Here's how the part is built. I have some questions about the finished solid (model axes, mm). A direction names the side the tool comes from. Coordinates: 2 decimals unless noted, no trailing zeros. Write each loop counter-clockwise with the first axis right and the second up, starting at its lowest first coordinate (ties: lowest second). Pieces come first, ordered by that corner, then holes. Notation, with made-up numbers: (31, -1.5) -> (88, -1.5) arc R4 cw to (88, 4.5) -> close; hole circle Ø1 at (-3, 10.25). An arc over 180 degrees is marked (long way). Use a Markdown table: item, result. Add a question column.
```python
from build123d import *

# Parameters (mm, degrees)
F1_DEPTH    = 6.35
F3_DEPTH    = 38.1
F4_R        = 5.08
F5_T1_DEPTH = 52.07
F5_S5_W     = 5.08
F5_S5_H     = 5.08
F5_T6_DEPTH = 5.08


# Not quite as in the source:
# - a fillet or chamfer that OpenCascade refuses, or shapes differently, is made with other operations: its cross-section is extruded or revolved along the edge and cut away or added


with BuildPart() as f1:
    # F0 (on Top) → F1 (new body)
    with BuildSketch(Plane.XY):
        Polygon((69.2906975746, 0), (0, 0), (0, -69.8406398296), (38.6781543493, -69.8406398296), (38.6781543493, -35.7452183962), (69.2906975746, -35.7452183962), align=None)
    extrude(amount=F1_DEPTH)

    # F2 (on face) → F3 (join)
    with BuildSketch(Plane(origin=(0, 0, 0), x_dir=(1, 0, 0), z_dir=(0, 0, -1))):
        Polygon((5.08, 69.8406398296), (0, 69.8406398296), (0, 0), (69.2906975746, 0), (69.2906975746, 5.08), (5.08, 5.08), align=None)
    extrude(amount=F3_DEPTH)

    # F4
    f4_edges = [f1.edges().sort_by_distance(p)[0] for p in [
        (34.645349, 0, 6.35),
        (0, -34.92032, 6.35),
        (19.339077, -69.84064, 6.35),
        (38.678154, -52.792929, 6.35),
        (53.984426, -35.745218, 6.35),
        (69.290698, -17.872609, 6.35),
    ]]
    fillet(f4_edges, radius=F4_R)

    # F5: fillet of radius 5.08 on 1 edges, made by hand

    # F5_s2 → F5_t1 (cut)
    with BuildSketch(Plane.XY.offset(-50.8)):
        with BuildLine():
            ThreePointArc((5.08, 0), (1.4878975516, -1.4878975516), (0, -5.08))
            Line((0, -5.08), (0, 0))
            Line((0, 0), (5.08, 0))
        make_face()
    extrude(amount=F5_T1_DEPTH, mode=Mode.SUBTRACT)


with BuildPart() as f5_tool4:
    # F5_s5 → F5_t6 (new body)
    with BuildSketch(Plane.XZ.offset(5.08)):
        with Locations((2.54, 3.81)):
            Rectangle(F5_S5_W, F5_S5_H)
    extrude(amount=-F5_T6_DEPTH)

    # F5_s7 → F5_t8 (revolve, cut)
    with BuildSketch(Plane(origin=(5.08, -5.08, 1.27), x_dir=(0.7071067812, 0, -0.7071067812), z_dir=(0.7071067812, 0, 0.7071067812))):
        with BuildLine():
            ThreePointArc((0, -5.08), (5.08, 0), (0, 5.08))
            Line((0, 5.08), (0, -5.08))
        make_face()
    revolve(axis=Axis((5.08, -5.08, 1.27), (0, 1, 0)), mode=Mode.SUBTRACT)


with BuildPart() as f1_1:
    add(f1.part)

    # F5_t3: cut F5_tool4
    add(f5_tool4.part, mode=Mode.SUBTRACT)


solid = f1_1.part
```
Q1. Will these pins go through, and if not, where does the flat tip stop? pin 1 (19 mm diameter, centred on x = 36, z = -26.5, fed in from -Y); pin 2 (6 mm diameter, centred on y = -26, z = -17.5, fed in from -X); pin 3 (0.6 mm diameter, centred on x = 53.5, z = 1, fed in from -Y); pin 4 (19 mm diameter, centred on y = -52, z = -14.5, fed in from +X).
Q2. Suppose I cut it at C-C, the plane z = -10. Write out the boundary of the cut face in (x, y).
Q3. Suppose I cut it at D-D, the plane x = 37.5. Write out the boundary of the cut face in (y, z).
Q4. Suppose I cut it at B-B, the plane x = 6.5. Write out the boundary of the cut face in (y, z), and give its area (3 significant figures).
Q5. Which directions (+Z, -Z, +X, -X, +Y, -Y) give clear straight access to the entire face, cutting with the end or side of a thin tool? Please do faces 1 (the cylindrical face through (37.23, -49.98, 4.82)), 2 (the cylindrical face through (67.842, -17.622, 4.822)), 3 (the flat face through (30, -30, 0)).
Q6. Suppose I cut it at A-A, the plane y = -15. Write out the boundary of the cut face in (x, z), and give its area (3 significant figures).
Q7. Please list where these lines run through material, in increasing order: line 1 (Z direction, x = 39, y = -10.5); line 2 (X direction, y = -16, z = -15); line 3 (Y direction, x = 53.5, z = -31).
Answer key:
| question | item | result |
|---|---|---|
| 1 | pin 1 | stops at y = -5.08 |
| 1 | pin 2 | stops at x = 0 |
| 1 | pin 3 | stops at y = -35.75 |
| 1 | pin 4 | stops at x = 5.08 |
| 2 | outline | (0, -69.84) -> (5.08, -69.84) -> (5.08, -5.08) -> (69.29, -5.08) -> (69.29, 0) -> (5.08, 0) arc R5.08 ccw to (0, -5.08) -> close |
| 3 | outline | (-69.84, 0) -> (-5.08, 0) -> (-5.08, -38.1) -> (0, -38.1) -> (0, 1.27) arc R5.08 ccw to (-5.08, 6.35) -> (-30.67, 6.35) arc R5.08 ccw to (-34.57, 4.52) -> (-68.66, 4.52) arc R5.08 ccw to (-69.84, 1.27) -> close |
| 4 | outline | (-69.84, 0) -> (-5.08, 0) -> (-5.08, -38.1) -> (0, -38.1) -> (0, 1.27) arc R5.08 ccw to (-5.08, 6.35) -> (-64.76, 6.35) arc R5.08 ccw to (-69.84, 1.27) -> close |
| 4 | area | 626 mm^2 |
| 5 | face 1 | +Z, +X, -Y |
| 5 | face 2 | +Z, +X, +Y, -Y |
| 5 | face 3 | -Z, +X, -Y |
| 6 | outline | (0, -38.1) -> (5.08, -38.1) -> (5.08, 0) -> (69.29, 0) -> (69.29, 1.27) arc R5.08 ccw to (64.21, 6.35) -> (5.08, 6.35) arc R5.08 ccw to (0, 1.27) -> close |
| 6 | area | 622 mm^2 |
| 7 | line 1 | z = 0 to 6.35 |
| 7 | line 2 | x = 0 to 5.08 |
| 7 | line 3 | y = -5.08 to 0 |
